Here's how the part is built. I have some questions about the finished solid (model axes, mm). A direction names the side the tool comes from. Give positions to 0.01 mm unless a question says otherwise; leave off trailing zeros. Use one line per item in the form item = value.
from build123d import *

# Parameters (mm, degrees)
F1_DEPTH      = 31
F1_DEPTH_BACK = 31
F2_R          = 25
F2_R_2        = 3
F3_DEPTH      = 6
F4_COUNT      = 8
F5_COUNT      = 2
F5_ANGLE      = 90
F6_COUNT      = 2
F6_ANGLE      = 90
F7_DEPTH      = 180.6822408671
F8_DEPTH      = 149.6822408671
F9_DEPTH      = 180.6822408671
F10_DEPTH     = 149.6822408671
F11_DEPTH     = 180.6822408671
F12_DEPTH     = 149.6822408671
F13_DEPTH     = 180.6822408671
F14_DEPTH     = 180.6822408671
F15_DEPTH     = 180.6822408671


with BuildPart() as f1:
    # F0 (on Front) → F1 (new body, two sides)
    with BuildSketch(Plane.XZ) as f1_sk:
        Polygon((74.8406204336, 31), (0, 31), (0, 0), (0, -31), (74.8406204336, -31), (74.8406204336, 0), align=None)
    extrude(amount=F1_DEPTH)
    extrude(f1_sk.sketch, amount=-F1_DEPTH_BACK)

    # F2 (on face) → F3 (cut)
    with BuildSketch(Plane.YZ.offset(74.8406204336)):
        Circle(F2_R)
        Circle(F2_R_2, mode=Mode.SUBTRACT)
    extrude(amount=-F3_DEPTH, mode=Mode.SUBTRACT)

    # F4: F1 ×8 about axis
    f4_axis = Axis((0, 0, 15.5), (0, 0, 1))


with BuildPart() as f1_1:
    add(f1.part)
    for i in range(1, F4_COUNT):
        add(f1.part.rotate(f4_axis, i * 360 / F4_COUNT))

    # F5: F1 ×2 about axis
    f5_axis = Axis((15.5, 0, 0), (1, 0, 0))


with BuildPart() as f1_2:
    add(f1_1.part)
    for i in range(1, F5_COUNT):
        add(f1_1.part.rotate(f5_axis, i * F5_ANGLE / (F5_COUNT - 1)))

    # F6: F1 ×2 about axis
    f6_axis = Axis((0, 0, 15.5), (0, 0, 1))


with BuildPart() as f1_3:
    add(f1_2.part)
    for i in range(1, F6_COUNT):
        add(f1_2.part.rotate(f6_axis, i * F6_ANGLE / (F6_COUNT - 1)))

    # F7 (cut, through all): a face of the model
    f7_faces = [f1_3.faces().sort_by_distance(p)[0] for p in [
        (-52.9203102168, -52.9203102168, 0),
    ]]
    extrude(f7_faces, amount=-F7_DEPTH, mode=Mode.SUBTRACT)

    # F8 (cut, through all): a face of the model
    f8_faces = [f1_3.faces().sort_by_distance(p)[0] for p in [
        (0, 74.8406204336, 0),
    ]]
    extrude(f8_faces, amount=-F8_DEPTH, mode=Mode.SUBTRACT)

    # F9 (cut, through all): a face of the model
    f9_faces = [f1_3.faces().sort_by_distance(p)[0] for p in [
        (-52.9203102168, 52.9203102168, 0),
    ]]
    extrude(f9_faces, amount=-F9_DEPTH, mode=Mode.SUBTRACT)

    # F10 (cut, through all): a face of the model
    f10_faces = [f1_3.faces().sort_by_distance(p)[0] for p in [
        (-74.8406204336, 0, 0),
    ]]
    extrude(f10_faces, amount=-F10_DEPTH, mode=Mode.SUBTRACT)

    # F11 (cut, through all): a face of the model
    f11_faces = [f1_3.faces().sort_by_distance(p)[0] for p in [
        (-52.9203102168, 0, -52.9203102168),
    ]]
    extrude(f11_faces, amount=-F11_DEPTH, mode=Mode.SUBTRACT)

    # F12 (cut, through all): a face of the model
    f12_faces = [f1_3.faces().sort_by_distance(p)[0] for p in [
        (0, 0, -74.8406204336),
    ]]
    extrude(f12_faces, amount=-F12_DEPTH, mode=Mode.SUBTRACT)

    # F13 (cut, through all): a face of the model
    f13_faces = [f1_3.faces().sort_by_distance(p)[0] for p in [
        (52.9203102168, 0, -52.9203102168),
    ]]
    extrude(f13_faces, amount=-F13_DEPTH, mode=Mode.SUBTRACT)

    # F14 (cut, through all): a face of the model
    f14_faces = [f1_3.faces().sort_by_distance(p)[0] for p in [
        (0, 52.9203102168, -52.9203102168),
    ]]
    extrude(f14_faces, amount=-F14_DEPTH, mode=Mode.SUBTRACT)

    # F15 (cut, through all): a face of the model
    f15_faces = [f1_3.faces().sort_by_distance(p)[0] for p in [
        (0, 52.9203102168, 52.9203102168),
    ]]
    extrude(f15_faces, amount=-F15_DEPTH, mode=Mode.SUBTRACT)


solid = f1_3.part
(1) Thinking about a two-plate mould opening in Z: for faces 5 (the cylindrical face through (36.53, 0.65, 2.93)), 6 (the flat face through (-21.1, 62.97, 42.87)), 7 (the flat face through (-14, 21, -74.841)), 8 (the flat face through (-31, 43, 43)), which applies, pulls with the +Z half, pulls with the -Z half, needs draft (parallel to the pull), parting line crosses it, or undercut?
Geometry says:
face_5 = undercut
face_6 = pulls with the +Z half
face_7 = pulls with the -Z half
face_8 = needs draft
(2) For faces 1 (the flat face through (0.35, -44.997, -52.359)), 2 (the cylindrical face through (71.883, 23.846, 7.509)), 3 (the flat face through (48, -48, -31)), 4 (the cylindrical face through (23.846, -7.509, -71.883)), which set-ups out of +Z, -Z, +X, -X, +Y, -Y let a thin tool reach every point of the face, with its end or its side?
Geometry says:
face_1 = none
face_2 = +X
face_3 = -Z, +X, -Y
face_4 = -Z
(3) For P1, Ø7, axis at x = 0, z = 0, coming from the +Y side; P2, Ø22, axis at x = -54, z = -53.5, coming from the -Y side; P3, Ø8, axis at y = -8.5, z = 22, coming from the -X side; P4, Ø2, axis at y = -57, z = 1.5, coming from the +X side, each with a flat end and sliding along its axis, tell me the tip position at first contact or that it passes through.
Geometry says:
P1 = 68.84
P2 = -31
P3 = -74.84
P4 = 41.36
(4) If we section it at A-A (z = 0): Give the number of separate pieces and of enclosed holes in the cut face, plus the area to 3 significant figures.
Geometry says:
separate_pieces = 8
enclosed_holes = 0
area = 13,000 mm²
(5) If I drill on probe 1 along X at (y, z) = (-24, 27); probe 2 along X at (y, z) = (17, 2.5); probe 3 along Z at (x, y) = (13.5, -0.5), over which ranges is the centre line in solid material (lowest first)?
Geometry says:
probe_1 = -74.84 to -2.12, 2.12 to 74.84
probe_2 = -68.84 to -19.35, -14.65 to -1.66, 1.66 to 14.65, 19.35 to 68.84
probe_3 = -68.84 to -17.68, -9.32 to -2.96, 2.96 to 9.32, 17.68 to 68.84
